```python
from build123d import *

# Parameters (mm, degrees)
SKETCH042_R     = 1.8
SKETCH042_R_2   = 16.2
SKETCH042_R_3   = 1.2
SKETCH042_R_4   = 1.5
PAD008_DEPTH    = 4
POCKET027_DEPTH = 1.2
SKETCH050_R     = 2
POCKET033_DEPTH = 1.2
POCKET033_TAPER = 45


with BuildPart() as part:
    # Sketch042 → Pad008 (new body)
    with BuildSketch(Plane.XY):
        with BuildLine():
            Line((35, 85), (35, -85))
            ThreePointArc((30, -90), (33.535534, -88.535534), (35, -85))
            Line((30, -90), (-52.963517, -90))
            ThreePointArc((-56.456955, -88.577135), (-54.849561, -89.630641), (-52.963517, -90))
            Line((-56.456955, -88.577135), (-143.493437, -3.577135))
            ThreePointArc((-143.493437, 3.577135), (-145, 0), (-143.493437, -3.577135))
            Line((-143.493437, 3.577135), (-56.456955, 88.577135))
            ThreePointArc((-52.963517, 90), (-54.849561, 89.630641), (-56.456955, 88.577135))
            Line((-52.963517, 90), (30, 90))
            ThreePointArc((35, 85), (33.535534, 88.535534), (30, 90))
        make_face()
        with Locations((-140, 0)):
            Circle(SKETCH042_R, mode=Mode.SUBTRACT)
        with Locations((30, -85)):
            Circle(SKETCH042_R, mode=Mode.SUBTRACT)
        with Locations((30, 85)):
            Circle(SKETCH042_R, mode=Mode.SUBTRACT)
        with Locations((-73.5, 0)):
            Circle(SKETCH042_R_2, mode=Mode.SUBTRACT)
        with Locations((-30, -38)):
            Circle(SKETCH042_R_3, mode=Mode.SUBTRACT)
        with Locations((-30, -52)):
            Circle(SKETCH042_R_3, mode=Mode.SUBTRACT)
        with Locations((-48.4, -38)):
            Circle(SKETCH042_R_3, mode=Mode.SUBTRACT)
        with Locations((-48.4, -52)):
            Circle(SKETCH042_R_3, mode=Mode.SUBTRACT)
        with Locations((0, 28)):
            Circle(SKETCH042_R_4, mode=Mode.SUBTRACT)
        with Locations((0, -28)):
            Circle(SKETCH042_R_4, mode=Mode.SUBTRACT)
        with Locations((-70, 20)):
            Circle(SKETCH042_R_4, mode=Mode.SUBTRACT)
        with Locations((-70, -20)):
            Circle(SKETCH042_R_4, mode=Mode.SUBTRACT)
        with Locations((-52.963517, -85)):
            Circle(SKETCH042_R, mode=Mode.SUBTRACT)
        with Locations((-52.963517, 85)):
            Circle(SKETCH042_R, mode=Mode.SUBTRACT)
        with BuildLine():
            Line((-56.5, 23.5), (-56.5, -23.5))
            ThreePointArc((-56.5, -23.5), (-55.035534, -27.035534), (-51.5, -28.5))
            Line((-51.5, -28.5), (-15.5, -28.5))
            ThreePointArc((-15.5, -28.5), (-11.964466, -27.035534), (-10.5, -23.5))
            Line((-10.5, -23.5), (-10.5, 23.5))
            ThreePointArc((-10.5, 23.5), (-11.964466, 27.035534), (-15.5, 28.5))
            Line((-15.5, 28.5), (-51.5, 28.5))
            ThreePointArc((-51.5, 28.5), (-55.035534, 27.035534), (-56.5, 23.5))
        make_face(mode=Mode.SUBTRACT)
        with BuildLine():
            Line((22, -30), (26, -30))
            ThreePointArc((30, -34), (28.828427, -31.171573), (26, -30))
            Line((30, -34), (30, -68))
            ThreePointArc((26, -72), (28.828427, -70.828427), (30, -68))
            Line((26, -72), (-52.963517, -72))
            ThreePointArc((-55.758267, -70.861708), (-54.472353, -71.704513), (-52.963517, -72))
            Line((-55.758267, -70.861708), (-90.57286, -36.861708))
            ThreePointArc((-87.77811, -30), (-91.482623, -32.491165), (-90.57286, -36.861708))
            Line((-87.77811, -30), (-82.820454, -30))
            ThreePointArc((-80.025704, -31.138292), (-81.311619, -30.295487), (-82.820454, -30))
            Line((-80.025704, -31.138292), (-51.638073, -58.861708))
            ThreePointArc((-51.638073, -58.861708), (-50.352158, -59.704513), (-48.843323, -60))
            Line((-48.843323, -60), (14, -60))
            ThreePointArc((14, -60), (16.828427, -58.828427), (18, -56))
            Line((18, -56), (18, -34))
            ThreePointArc((22, -30), (19.171573, -31.171573), (18, -34))
        make_face(mode=Mode.SUBTRACT)
        with BuildLine():
            Line((22, 10), (26, 10))
            ThreePointArc((26, 10), (28.828427, 11.171573), (30, 14))
            Line((30, 14), (30, 68))
            ThreePointArc((30, 68), (28.828427, 70.828427), (26, 72))
            Line((26, 72), (-52.963517, 72))
            ThreePointArc((-52.963517, 72), (-54.472353, 71.704513), (-55.758267, 70.861708))
            Line((-55.758267, 70.861708), (-84.375349, 42.91421))
            ThreePointArc((-84.375349, 42.91421), (-85.285112, 38.543667), (-81.580599, 36.052502))
            Line((-81.580599, 36.052502), (-76.622942, 36.052502))
            ThreePointArc((-76.622942, 36.052502), (-75.114107, 36.347989), (-73.828192, 37.190794))
            Line((-73.828192, 37.190794), (-51.638073, 58.861708))
            ThreePointArc((-48.843323, 60), (-50.352158, 59.704513), (-51.638073, 58.861708))
            Line((-48.843323, 60), (14, 60))
            ThreePointArc((18, 56), (16.828427, 58.828427), (14, 60))
            Line((18, 56), (18, 14))
            ThreePointArc((18, 14), (19.171573, 11.171573), (22, 10))
        make_face(mode=Mode.SUBTRACT)
        with BuildLine():
            Line((-97.128995, -24.026251), (-102.086655, -24.026251))
            ThreePointArc((-104.881405, -22.887959), (-103.59549, -23.730764), (-102.086655, -24.026251))
            Line((-104.881405, -22.887959), (-125.387457, -2.861708))
            ThreePointArc((-125.387457, 2.861708), (-126.592707, 0), (-125.387457, -2.861708))
            Line((-125.387457, 2.861708), (-104.881397, 22.887967))
            ThreePointArc((-102.086647, 24.026259), (-103.595482, 23.730772), (-104.881397, 22.887967))
            Line((-102.086647, 24.026259), (-97.128986, 24.026259))
            ThreePointArc((-94.334245, 17.164543), (-93.424471, 21.535089), (-97.128986, 24.026259))
            Line((-106.049485, 5.723416), (-94.334245, 17.164543))
            ThreePointArc((-106.049485, 5.723416), (-106.941129, 4.414287), (-107.254735, 2.861708))
            Line((-107.254735, -2.861708), (-107.254735, 2.861708))
            ThreePointArc((-107.254735, -2.861708), (-106.941129, -4.414287), (-106.049485, -5.723416))
            Line((-94.334245, -17.164543), (-106.049485, -5.723416))
            ThreePointArc((-97.128995, -24.026251), (-93.424482, -21.535086), (-94.334245, -17.164543))
        make_face(mode=Mode.SUBTRACT)
        with BuildLine():
            Line((-22.4, -38), (-22.4, -52))
            ThreePointArc((-22.4, -52), (-21.228427, -54.828427), (-18.4, -56))
            Line((-18.4, -56), (0, -56))
            ThreePointArc((0, -56), (2.828427, -54.828427), (4, -52))
            Line((4, -52), (4, -38))
            ThreePointArc((4, -38), (2.828427, -35.171573), (0, -34))
            Line((0, -34), (-18.4, -34))
            ThreePointArc((-18.4, -34), (-21.228427, -35.171573), (-22.4, -38))
        make_face(mode=Mode.SUBTRACT)
    extrude(amount=PAD008_DEPTH)

    # Sketch043 (on Face87 of Pad008) → Pocket027 (cut)
    with BuildSketch(Plane(origin=(0, 0, 0), x_dir=(1, 0, 0), z_dir=(0, 0, -1))):
        Polygon((-136.6, 0), (-138.3, 2.944486), (-141.7, 2.944486), (-143.4, 0), (-141.7, -2.944486), (-138.3, -2.944486), align=None)
        Polygon((30, -81.6), (27.055514, -83.3), (27.055514, -86.7), (30, -88.4), (32.944486, -86.7), (32.944486, -83.3), align=None)
        Polygon((30, 81.6), (32.944486, 83.3), (32.944486, 86.7), (30, 88.4), (27.055514, 86.7), (27.055514, 83.3), align=None)
        Polygon((-67.401924, 18.5), (-67.401924, 21.5), (-70, 23), (-72.598076, 21.5), (-72.598076, 18.5), (-70, 17), align=None)
        Polygon((-67.401924, -21.5), (-67.401924, -18.5), (-70, -17), (-72.598076, -18.5), (-72.598076, -21.5), (-70, -23), align=None)
        Polygon((0, 25), (2.598076, 26.5), (2.598076, 29.5), (0, 31), (-2.598076, 29.5), (-2.598076, 26.5), align=None)
        Polygon((2.598076, -29.5), (2.598076, -26.5), (0, -25), (-2.598076, -26.5), (-2.598076, -29.5), (0, -31), align=None)
        Polygon((-52.963517, -81.6), (-55.908004, -83.3), (-55.908004, -86.7), (-52.963517, -88.4), (-50.019031, -86.7), (-50.019031, -83.3), align=None)
        Polygon((-52.963517, 81.6), (-50.019031, 83.3), (-50.019031, 86.7), (-52.963517, 88.4), (-55.908004, 86.7), (-55.908004, 83.3), align=None)
    extrude(amount=-POCKET027_DEPTH, mode=Mode.SUBTRACT)

    # Sketch050 (on Face4 of Pocket027) → Pocket033 (cut)
    with BuildSketch(Plane(origin=(0, 0, 0), x_dir=(1, 0, 0), z_dir=(0, 0, -1))):
        with Locations((-48.4, 52)):
            Circle(SKETCH050_R)
        with Locations((-48.4, 38)):
            Circle(SKETCH050_R)
        with Locations((-30, 38)):
            Circle(SKETCH050_R)
        with Locations((-30, 52)):
            Circle(SKETCH050_R)
    extrude(amount=-POCKET033_DEPTH, taper=POCKET033_TAPER, mode=Mode.SUBTRACT)


with BuildPart() as part_1:
    # Body005 placement: moved
    add(part.part.moved(Location((0, 0, 100))))


solid = part_1.part
```
Model file for the job. Use its own axes, mm. A direction names the side the tool comes from. Give positions to 0.01 mm unless a question says otherwise; leave off trailing zeros. Order: outer loops, then holes, each group sorted by start corner. A loop starts at its lowest first (then second) coordinate and runs counter-clockwise, first axis right, second up.
1) 3-axis set-ups, long thin cutter, end or side, ignore diameter. For faces 1 (the flat face through (-71.2, -18.7, 101.2)), 2 (the flat face through (-22.4, -45, 102)): which of +Z, -Z, +X, -X, +Y, -Y reach the whole face in a straight line?
2) Saw through at A-A, the plane x = -35. Write the cut outline in (y, z).
3) Wall check: probe 1 along Y at (x, z) = (0, 102.7); probe 2 along X at (y, z) = (-85, 102.9); probe 3 along X at (y, z) = (-28, 102.95). Give the ranges that are in metal, low to high.
4) Pin check, flat tips, straight feed: pin 1 (1.5 mm diameter, centred on y = 56, z = 100.5, fed in from -X); pin 2 (4.5 mm diameter, centred on x = -140, y = 0, fed in from -Z); pin 3 (1.3 mm diameter, centred on y = 85.5, z = 100.5, fed in from +X); pin 4 (1 mm diameter, centred on y = 20, z = 100.5, fed in from -X). Stop position of each tip, or through.
5) Saw through at C-C, the plane y = 64.5. Write the cut outline in (x, z).
6) Mould opens along X. For faces 3 (the flat face through (-18, 60, 102)), 4 (the flat face through (-34, -39, 104)), 5 (the flat face through (-69.87, 57.08, 101.97)) say: +X half, -X half, draft (parallel to the pull), parting line (faces both ways), or undercut.
7) Saw through at B-B, the plane y = -44.5. Write the cut outline in (x, z).
Computed:
1. face 1: -Z
1. face 2: +Z, -Z
2. outline: (-90, 100) - (-72, 100) - (-72, 104) - (-90, 104) - close; (-60, 100) - (-28.5, 100) - (-28.5, 104) - (-60, 104) - close; (28.5, 100) - (60, 100) - (60, 104) - (28.5, 104) - close; (72, 100) - (90, 100) - (90, 104) - (72, 104) - close
3. probe 1: y = -90 to -72, -60 to -56, -34 to -29.5, -26.5 to 26.5, 29.5 to 60, 72 to 90
3. probe 2: x = -60.12 to -54.76, -51.16 to 28.2, 31.8 to 35
3. probe 3: x = -118.49 to -53.68, -13.32 to -1.5, 1.5 to 35
4. pin 1: stops at x = -90.58
4. pin 2: stops at z = 101.2
4. pin 3: stops at x = 35
4. pin 4: stops at x = -127.19
5. outline: (-81.11, 100) - (-62.27, 100) - (-62.27, 104) - (-81.11, 104) - close; (30, 100) - (35, 100) - (35, 104) - (30, 104) - close
6. face 3: undercut
6. face 4: draft
6. face 5: undercut
7. outline: (-101.59, 100) - (-82.75, 100) - (-82.75, 104) - (-101.59, 104) - close; (-66.34, 100) - (-22.4, 100) - (-22.4, 104) - (-66.34, 104) - close; (4, 100) - (18, 100) - (18, 104) - (4, 104) - close; (30, 100) - (35, 100) - (35, 104) - (30, 104) - close
